Input: dimensioned drawing with shaded views. Units: mm. Origin: part minimum x, y, z. A direction names the side the tool comes from. Round coordinates to 2 decimals unless told otherwise and drop trailing zeros. Loops run counter-clockwise (first coordinate to the right, second up) from the corner with the lowest first, then second, coordinate; pieces in that order, holes last. Notation, with made-up numbers: M 87,-30.75 L 135,-30.75 A23 ccw 135,3.25 Z; hole C 63,12 d5. An arc over 180 degrees is marked long. One line per item, written item: value.
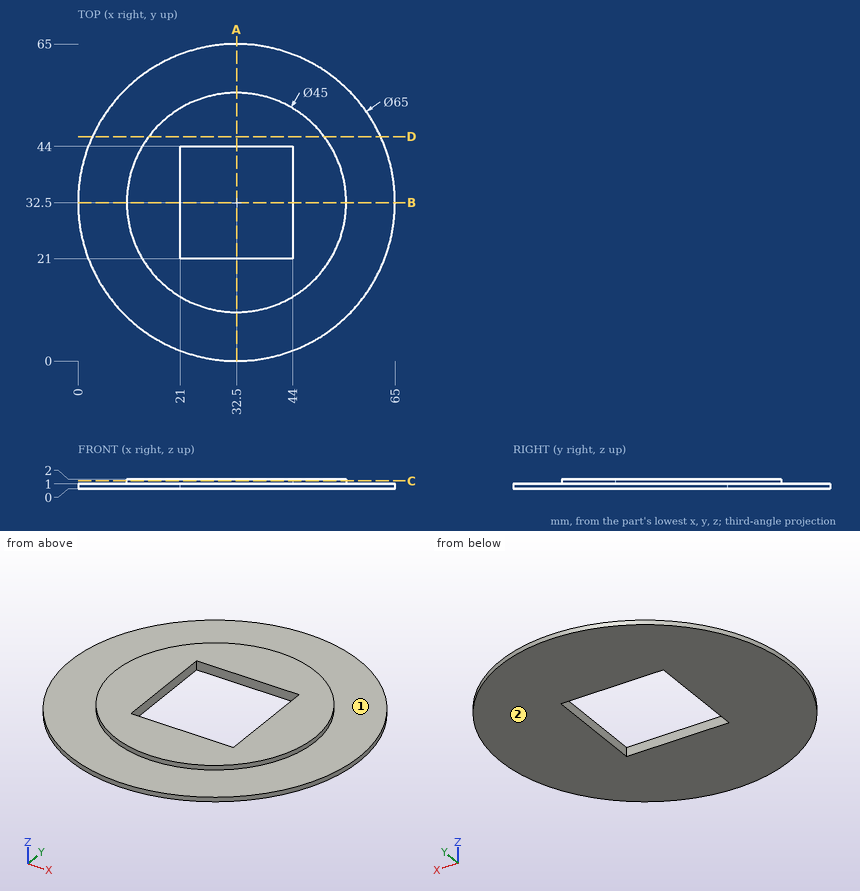
1. Section query C-C (z = 1.6). Return the cut outline in (x, y).
Report:
outline: C 32.5,32.5 d45; hole M 21,21 L 44,21 L 44,44 L 21,44 Z
2. Section query D-D (y = 46). Return the cut outline in (x, z), and give its area (3 significant figures).
Report:
outline: M 2.94,0 L 62.06,0 L 62.06,1 L 50.5,1 L 50.5,2 L 14.5,2 L 14.5,1 L 2.94,1 Z
area: 95.1 mm2
3. Reachability of the marked faces 1 and 2 from +Z, -Z, +X, -X, +Y, -Y: full face, straight path, thin tool, end or side. Return the list, or none.
Report:
face 1: +Z
face 2: -Z, +X, -X, +Y, -Y
4. Pin query (flat end, axial travel): pin 1 (19.5 mm diameter, centred on x = 26.5, y = 41.5, fed in from +Z); pin 2 (1 mm diameter, centred on y = 24, z = 0.5, fed in from -X). Return the tip coordinate at first contact, or that it passes through.
Report:
pin 1: stops at z = 2
pin 2: stops at x = 1
5. Section query A-A (x = 32.5). Return the cut outline in (y, z).
Report:
outline: M 0,0 L 21,0 L 21,2 L 10,2 L 10,1 L 0,1 Z; M 44,0 L 65,0 L 65,1 L 55,1 L 55,2 L 44,2 Z
6. Ray query, line 1 (X direction, y = 28, z = 1.5); line 2 (X direction, y = 40, z = 1.25); line 3 (Z direction, x = 21, y = 6.5). Return the intervals inside material, ascending. Write a range as [from, to].
Report:
line 1: x = [10.45, 21], [44, 54.55]
line 2: x = [11.29, 21], [44, 53.71]
line 3: z = [0, 1]
